Here's how the part is built. I have some questions about the finished solid (model axes, mm). Face numbers are marked on the shaded views. A direction names the side the tool comes from. Give positions to 0.01 mm unless a question says otherwise; leave off trailing zeros. Write each loop counter-clockwise with the first axis right and the second up, starting at its lowest first coordinate (ties: lowest second). Pieces come first, ordered by that corner, then holes. Notation, with made-up numbers: (38.25, 31) -> (85.25, 31) arc R36 ccw to (85.25, 65) -> close; hole circle Ø8 at (17.5, -18). An arc over 180 degrees is marked (long way). Use CSV: the item, a comma, the result in double quotes. Start each with the question number.
(1) For pin 1 Ø1.5 at (x, y) = (0.5, -3.5) entering from -Z; pin 2 Ø1 at (y, z) = (-3, -6.5) entering from +X; pin 3 Ø6 at (y, z) = (-0.5, -16.5) entering from +X, each with a flat end and sliding along its axis, tell me the tip position at first contact or that it passes through.
(2) Suppose I cut it at B-B on x = 0. List the corners of the cut face in (y, z) for me.
(3) Suppose I cut it at A-A on z = -30.5. List the corners of the cut face in (x, y) for me, plus the area to 3 significant figures.
(4) Suppose I cut it at C-C on x = -3.5. List the corners of the cut face in (y, z) for me, plus the area to 3 significant figures.
(5) I need wall thicknesses on L1, parallel to Y at x = 0, z = 11.5; L2, parallel to Z at x = -5, y = 0.5; L3, parallel to Z at x = 3, y = 1. Which ranges of each line are inside material? Lowest first, please. Write a range as [from, to].
(6) Which directions (+Z, -Z, +X, -X, +Y, -Y) give clear straight access to the entire face, cutting with the end or side of a thin tool? Please do the marked faces 1, 2, 3 and 4.
from build123d import *

# Parameters (mm, degrees)
SKETCH1_R           = 6.35
BOSS_EXTRUDE1_DEPTH = 12.7
BOSS_EXTRUDE2_DEPTH = 38.1
SKETCH8_R           = 1.27
BOSS_EXTRUDE3_DEPTH = 5.08
CUT_EXTRUDE1_DEPTH  = 13.97
SKETCH10_R          = 1.27
CUT_EXTRUDE2_DEPTH  = 5.08
SKETCH11_R          = 2
CUT_EXTRUDE3_DEPTH  = 6.35


with BuildPart() as part:
    # Sketch1 → Boss-Extrude1 (new body)
    with BuildSketch(Plane.XY):
        Circle(SKETCH1_R)
    extrude(amount=BOSS_EXTRUDE1_DEPTH)

    # Sketch3 → Boss-Extrude2 (add)
    with BuildSketch(Plane(origin=(0, 0, 0), x_dir=(-1, 0, 0), z_dir=(0, 0, -1))):
        Polygon((0.489155942, 3.00848222), (-2.360844058, 1.927862582), (-2.85, -1.080619638), (-0.489155942, -3.00848222), (2.360844058, -1.927862582), (2.85, 1.080619638), align=None)
    extrude(amount=BOSS_EXTRUDE2_DEPTH)

    # Sketch8 → Boss-Extrude3 (add)
    with BuildSketch(Plane(origin=(0, 0, -38.1), x_dir=(-1, 0, 0), z_dir=(0, 0, -1))):
        Circle(SKETCH8_R)
    extrude(amount=BOSS_EXTRUDE3_DEPTH)

    # Sketch9 → Cut-Extrude1 (cut)
    with BuildSketch(Plane(origin=(0, 0, 0), x_dir=(-1, 0, 0), z_dir=(0, 0, -1))):
        Polygon((-5.082038886, -3.807279968), (-3.718493538, 5.14735911), (-6.16534328, 5.519947057), (-7.528888629, -3.434692022), align=None)
    extrude(amount=-CUT_EXTRUDE1_DEPTH, mode=Mode.SUBTRACT)

    # Sketch10 → Cut-Extrude2 (cut)
    with BuildSketch(Plane(origin=(4.400266212, 0.670039571, 0), x_dir=(0, 0, -1), z_dir=(0.988604335884072, 0.1505372614046529, 0))):
        with Locations(Location((-9.446434999, 0, 0), (0, 0, 90))):
            Circle(SKETCH10_R)
    extrude(amount=-CUT_EXTRUDE2_DEPTH, mode=Mode.SUBTRACT)

    # Sketch11 → Cut-Extrude3 (cut)
    with BuildSketch(Plane.XY.offset(12.7)):
        Circle(SKETCH11_R)
    extrude(amount=-CUT_EXTRUDE3_DEPTH, mode=Mode.SUBTRACT)


solid = part.part
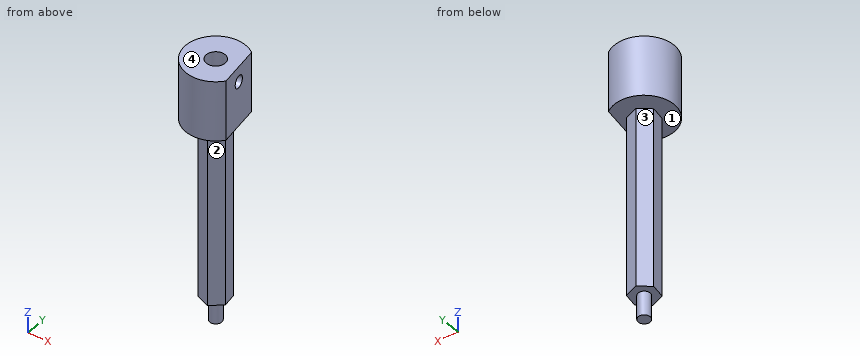
Geometry says:
1,pin 1,"z = -38.1"
1,pin 2,"x = 1.11"
1,pin 3,"x = 2.85"
2,outline,"(-6.35, 0) -> (-2.82, 0) -> (-2.82, -38.1) -> (-1.27, -38.1) -> (-1.27, -43.18) -> (1.27, -43.18) -> (1.27, -38.1) -> (2.82, -38.1) -> (2.82, 0) -> (6.35, 0) -> (6.35, 12.7) -> (2, 12.7) -> (2, 6.35) -> (-2, 6.35) -> (-2, 12.7) -> (-6.35, 12.7) -> close"
3,outline,"(-2.85, 1.08) -> (-2.36, -1.93) -> (0.49, -3.01) -> (2.85, -1.08) -> (2.36, 1.93) -> (-0.49, 3.01) -> close"
3,area,"24.1 mm²"
4,outline,"(-5.3, 0) -> (5.3, 0) -> (5.3, 12.7) -> (-5.3, 12.7) -> close"
4,area,"135 mm²"
5,L1,"[-6.35, -2], [2, 6.35]"
5,L2,"[0, 12.7]"
5,L3,"[0, 8.3], [10.6, 12.7]"
6,face 1,"-Z"
6,face 2,"-Z, +X, -Y"
6,face 3,"-Z, -X, +Y"
6,face 4,"+Z, +X, -X, +Y, -Y"
